from build123d import *

# Parameters (mm, degrees)
SKETCH1_W           = 54
SKETCH1_H           = 10
BOSS_EXTRUDE1_DEPTH = 90
SKETCH2_W           = 40.6
SKETCH2_H           = 19.8
CUT_EXTRUDE1_DEPTH  = 99.192875432
CUT_EXTRUDE2_DEPTH  = 99.192875432
BOSS_EXTRUDE4_DEPTH = 5
BOSS_EXTRUDE5_DEPTH = 5
SKETCH9_R           = 1
CUT_EXTRUDE3_DEPTH  = 108.549248187


with BuildPart() as part:
    # Sketch1 → Boss-Extrude1 (new body)
    with BuildSketch(Plane.XY):
        with Locations((10.971578656, 527.175634265)):
            Rectangle(SKETCH1_W, SKETCH1_H)
    extrude(amount=BOSS_EXTRUDE1_DEPTH)

    # Sketch2 → Cut-Extrude1 (cut, through all)
    with BuildSketch(Plane.XZ.offset(-522.175634265)):
        with Locations((10.971578656, 80.1)):
            Rectangle(SKETCH2_W, SKETCH2_H)
    extrude(amount=-CUT_EXTRUDE1_DEPTH, mode=Mode.SUBTRACT)

    # Sketch4 → Cut-Extrude2 (cut, through all)
    with BuildSketch(Plane(origin=(0, 532.175634265, 0), x_dir=(1, 0, 0), z_dir=(0, 1, 0))):
        with BuildLine():
            Line((7.971578656, -40), (7.971578656, 0))
            ThreePointArc((7.971578656, 0), (10.971578656, 3), (13.971578656, 0))
            Line((13.971578656, 0), (13.971578656, -40))
            ThreePointArc((13.971578656, -40), (10.971578656, -43), (7.971578656, -40))
        make_face()
    extrude(amount=-CUT_EXTRUDE2_DEPTH, mode=Mode.SUBTRACT)

    # Sketch7 → Boss-Extrude4 (add)
    with BuildSketch(Plane.ZY.offset(16.028421344)):
        Polygon((35, 532.175634265), (0, 567.175634265), (0, 532.175634265), align=None)
    extrude(amount=-BOSS_EXTRUDE4_DEPTH)

    # Sketch8 → Boss-Extrude5 (add)
    with BuildSketch(Plane(origin=(37.971578656, 0, 0), x_dir=(0, 0, -1), z_dir=(1, 0, 0))):
        Polygon((-35, 532.175634265), (0, 567.175634265), (0, 532.175634265), align=None)
    extrude(amount=-BOSS_EXTRUDE5_DEPTH)

    # Sketch9 → Cut-Extrude3 (cut, through all)
    with BuildSketch(Plane.XZ.offset(-522.175634265)):
        with Locations(Location((-13.228421344, 85.1, 0), (0, 0, 270))):
            Circle(SKETCH9_R)
        with Locations(Location((-13.228421344, 74.9, 0), (0, 0, 270))):
            Circle(SKETCH9_R)
        with Locations(Location((35.171578656, 74.9, 0), (0, 0, 270))):
            Circle(SKETCH9_R)
        with Locations(Location((35.171578656, 85.1, 0), (0, 0, 270))):
            Circle(SKETCH9_R)
    extrude(amount=-CUT_EXTRUDE3_DEPTH, mode=Mode.SUBTRACT)


solid = part.part
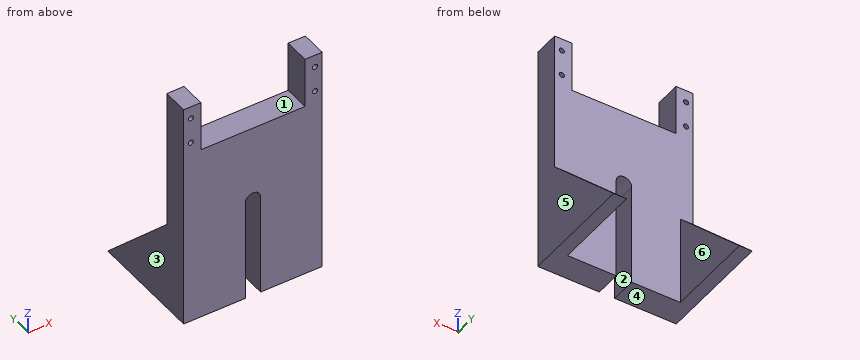
Work out the finished part from the listing and answer in its coordinate system (mm). Face numbers are marked on the shaded views. A direction names the side the tool comes from. Give positions to 0.01 mm unless a question says otherwise; leave off trailing zeros. Loops run counter-clockwise (first coordinate to the right, second up) from the corner with the lowest first, then second, coordinate; pieces in that order, holes last. Notation, with made-up numbers: (-36.5, -10) -> (-27.5, -10) arc R12 cw to (-27.5, -6) -> close; hole circle Ø1 at (76, -23). An arc over 180 degrees is marked (long way). Use a Markdown table: item, result. Add a question column.
1) The part is cut by section A-A, the plane z = 74.9. Determine the outline of the cut face in (x, y), plus the area to 3 significant figures.
2) Which of the six approach directions +Z, -Z, +X, -X, +Y, -Y give full straight-line access (tool end or side, diameter ignored) to the marked faces 1, 2 and 3?
3) For a pull along X with two mould halves and no side action, classify the marked faces 4, 5 and 6 as +X half, -X half, draft (parallel to the pull), parting line (faces both ways), or undercut.
4) The part is cut by section B-B, the plane y = 559. Determine the outline of the cut face in (x, z), plus the area to 3 significant figures.
5) Consider line 1 along X through (y, z) = (525.25, 74.9); line 2 along X through (y, z) = (536.5, 17.5); line 3 along X through (y, z) = (526.5, 81). Determine where each line is inside the solid, lowest interval first.
6) The part is cut by section D-D, the plane z = 48. Determine the outline of the cut face in (x, y), plus the area to 3 significant figures.
7) The part is cut by section C-C, the plane z = 11. Determine the outline of the cut face in (x, y).
8) Each of these flat-tipped pins is pushed along its axis until it touches: P1, Ø5, axis at x = 20, y = 528, coming from the +Z side; P2, Ø12, axis at x = 10.5, z = 56, coming from the +Y side. Where does it stop, or does it pass through?
Reported:
| question | item | result |
|---|---|---|
| 1 | outline | (-16.03, 522.18) -> (-14.23, 522.18) -> (-14.23, 532.18) -> (-16.03, 532.18) -> close; (-12.23, 522.18) -> (-9.33, 522.18) -> (-9.33, 532.18) -> (-12.23, 532.18) -> close; (31.27, 522.18) -> (34.17, 522.18) -> (34.17, 532.18) -> (31.27, 532.18) -> close; (36.17, 522.18) -> (37.97, 522.18) -> (37.97, 532.18) -> (36.17, 532.18) -> close |
| 1 | area | 94.0 mm^2 |
| 2 | face 1 | +Z, +Y, -Y |
| 2 | face 2 | -Z, +Y, -Y |
| 2 | face 3 | +Z, -Z, -X, +Y, -Y |
| 3 | face 4 | draft |
| 3 | face 5 | +X half |
| 3 | face 6 | undercut |
| 4 | outline | (-16.03, 0) -> (-11.03, 0) -> (-11.03, 8.18) -> (-16.03, 8.18) -> close; (32.97, 0) -> (37.97, 0) -> (37.97, 8.18) -> (32.97, 8.18) -> close |
| 4 | area | 81.8 mm^2 |
| 5 | line 1 | x = -16.03 to -14.23, -12.23 to -9.33, 31.27 to 34.17, 36.17 to 37.97 |
| 5 | line 2 | x = -16.03 to -11.03, 32.97 to 37.97 |
| 5 | line 3 | x = -16.03 to -9.33, 31.27 to 37.97 |
| 6 | outline | (-16.03, 522.18) -> (37.97, 522.18) -> (37.97, 532.18) -> (-16.03, 532.18) -> close |
| 6 | area | 540 mm^2 |
| 7 | outline | (-16.03, 522.18) -> (7.97, 522.18) -> (7.97, 532.18) -> (-11.03, 532.18) -> (-11.03, 556.18) -> (-16.03, 556.18) -> close; (13.97, 522.18) -> (37.97, 522.18) -> (37.97, 556.18) -> (32.97, 556.18) -> (32.97, 532.18) -> (13.97, 532.18) -> close |
| 8 | P1 | stops at z = 70.2 |
| 8 | P2 | stops at y = 532.18 |
